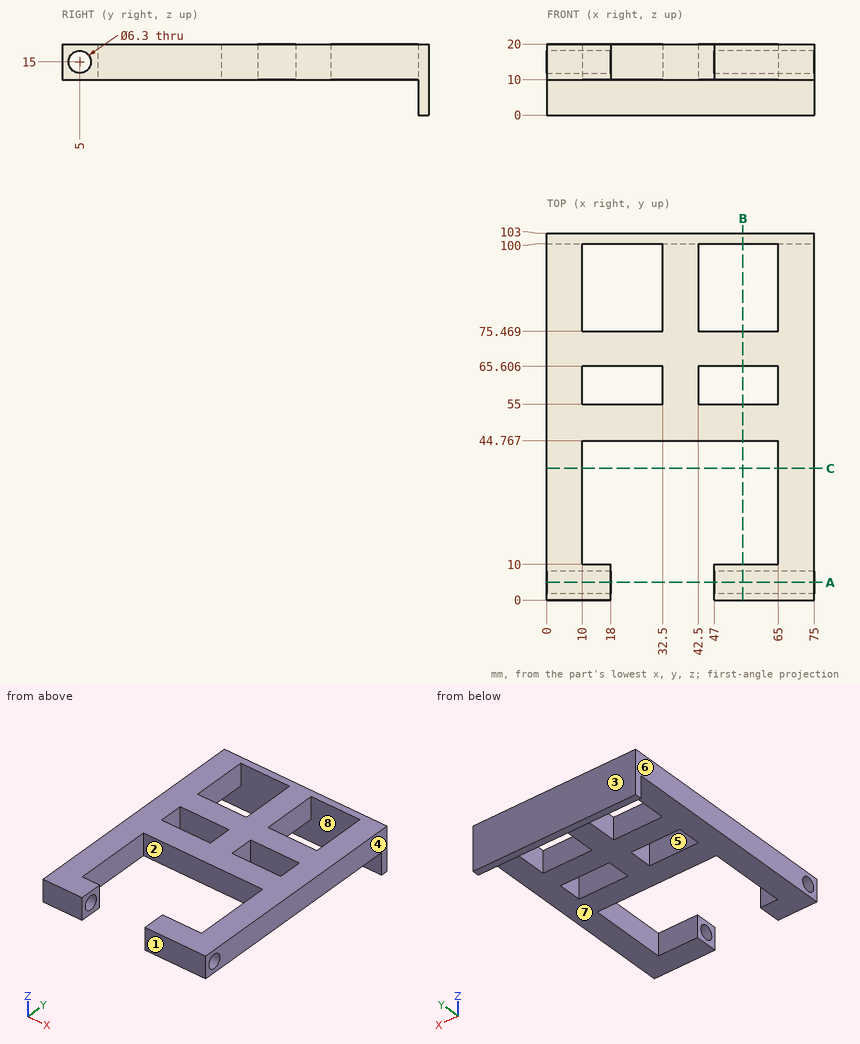
Source: three-view drawing plus pictorial views. Frame: mm from the lowest corner of the part. A direction names the side the tool comes from. Give positions to 0.01 mm unless a question says otherwise; leave off trailing zeros. Write each loop counter-clockwise with the first axis right and the second up, starting at its lowest first coordinate (ties: lowest second). Pieces come first, ordered by that corner, then holes. Notation, with made-up numbers: (35, 81) -> (88, 81) arc R5 ccw to (88, 87) -> close; hole circle Ø3 at (66, -32.5). An arc over 180 degrees is marked (long way). Answer in a Markdown table with one row per item.
(1) Section query B-B on x = 55. State how many separate pieces and enclosed holes the cut face has, then the cut area to 3 significant figures.
Answers below:
| item | result |
|---|---|
| separate pieces | 4 |
| enclosed holes | 1 |
| area | 330 mm^2 |
(2) Section query A-A on y = 5. Return loops of the section in (x, z).
Answers below:
| item | result |
|---|---|
| outline | (0, 10) -> (18, 10) -> (18, 11.85) -> (0, 11.85) -> close; (0, 18.15) -> (18, 18.15) -> (18, 20) -> (0, 20) -> close; (47, 10) -> (75, 10) -> (75, 11.85) -> (47, 11.85) -> close; (47, 18.15) -> (75, 18.15) -> (75, 20) -> (47, 20) -> close |
(3) Section query C-C on y = 37. Return loops of the section in (x, z), then the cut area to 3 significant figures.
Answers below:
| item | result |
|---|---|
| outline | (0, 10) -> (10, 10) -> (10, 20) -> (0, 20) -> close; (65, 10) -> (75, 10) -> (75, 20) -> (65, 20) -> close |
| area | 200 mm^2 |
(4) Ray query, line 1 along Y through (x, z) = (30, 15.25) (1 decimal); line 2 along Y through (x, z) = (57.5, 10.75) (1 decimal); line 3 along Y through (x, z) = (17.5, 16.5) (1 decimal). Return the intervals inside material, ascending. Write a range as [from, to].
Answers below:
| item | result |
|---|---|
| line 1 | [44.8, 55], [65.6, 75.5], [100, 103] |
| line 2 | [0, 10], [44.8, 55], [65.6, 75.5], [100, 103] |
| line 3 | [0, 2.2], [7.8, 10], [44.8, 55], [65.6, 75.5], [100, 103] |
(5) Pin query (flat end, axial travel): pin 1 (5 mm diameter, centred on y = 5, z = 14, fed in from -X); pin 2 (1 mm diameter, centred on x = 54.5, y = 74.5, fed in from -Z); pin 3 (11 mm diameter, centred on x = 32, z = 13.5, fed in from -Y). Return the tip coordinate at first contact, or that it passes through.
Answers below:
| item | result |
|---|---|
| pin 1 | x = 0 |
| pin 2 | z = 10 |
| pin 3 | y = 44.77 |
(6) Set-up query: the marked faces 5, 6, 7 and 8. Return all of +Z, -Z, +X, -X, +Y, -Y with unobstructed straight access to the full face (end or side cutting, diameter ignored); none if empty.
Answers below:
| item | result |
|---|---|
| face 5 | +Z, -Z |
| face 6 | +Z, -Z, -X, +Y, -Y |
| face 7 | -Z, +X, -X, -Y |
| face 8 | -Z |
(7) Draft query along Y for the marked faces 1, 2, 3 and 4. Return one class per face: +Y half, -Y half, draft (parallel to the pull), parting line (faces both ways), or undercut.
Answers below:
| item | result |
|---|---|
| face 1 | -Y half |
| face 2 | undercut |
| face 3 | +Y half |
| face 4 | draft |
